Read the model definition and answer for the solid it produces. Units are mm, in the model's axes. A direction names the side the tool comes from. Give positions to 0.01 mm unless a question says otherwise; leave off trailing zeros. Write each loop counter-clockwise with the first axis right and the second up, starting at its lowest first coordinate (ties: lowest second). Pieces come first, ordered by that corner, then holes. Notation, with made-up numbers: (-39, 6.25) -> (-32, 6.25) arc R24 ccw to (-32, 19.25) -> close; hole circle Ø1 at (12.25, 33). An arc over 180 degrees is marked (long way). Write item = value, one per line.
from build123d import *

# Parameters (mm, degrees)
BOSS_EXTRUDE1_DEPTH = 5
BOSS_EXTRUDE2_DEPTH = 5


with BuildPart() as part:
    # Sketch1 → Boss-Extrude1 (new body)
    with BuildSketch(Plane(origin=(0, 0, 0), x_dir=(1, 0, 0), z_dir=(0, 1, 0))):
        Polygon((-109.888174915, 15), (-130.65513844, 15), (-130.65513844, 0), (-102.893560042, 0), align=None)
        Polygon((-98.854395725, 15), (-109.888174915, 15), (-102.893560042, 0), (-91.859780853, 0), align=None)
        Polygon((-91.859780853, 15), (-98.854395725, 15), (-91.859780853, 0), (-84.86516598, 0), align=None)
        Polygon((-80.826001663, 15), (-91.859780853, 15), (-84.86516598, 0), (-73.831386791, 0), align=None)
        Polygon((1.48976704, 15), (-80.826001663, 15), (-73.831386791, 0), (1.48976704, 0), align=None)
    extrude(amount=-BOSS_EXTRUDE1_DEPTH)

    # Sketch1_3 → Boss-Extrude2 (add)
    with BuildSketch(Plane(origin=(0, 0, 0), x_dir=(1, 0, 0), z_dir=(0, 1, 0))):
        Polygon((-109.888174915, 15), (-130.65513844, 15), (-130.65513844, 0), (-102.893560042, 0), align=None)
        Polygon((-91.859780853, 15), (-98.854395725, 15), (-91.859780853, 0), (-84.86516598, 0), align=None)
        Polygon((1.48976704, 15), (-80.826001663, 15), (-73.831386791, 0), (1.48976704, 0), align=None)
    extrude(amount=BOSS_EXTRUDE2_DEPTH)


solid = part.part
(1) Consider L1, parallel to X at y = 2.25, z = -2.75; L2, parallel to X at y = 3.75, z = -0.75; L3, parallel to Y at x = -99, z = -13.75. Determine where each line is inside the solid, lowest interval first.
Checks:
L1 = -130.66 to -104.18, -93.14 to -86.15, -75.11 to 1.49
L2 = -130.66 to -103.24, -92.21 to -85.21, -74.18 to 1.49
L3 = -5 to 0
(2) A tool of negligible diameter and unlimited length cuts with its end or side. For faces 4 (the flat face through (-83, 0, -8)), 5 (the flat face through (-64, 0, -15)), 6 (the flat face through (-77.378, 2.465, -7.605)), 7 (the flat face through (-106.342, 2.465, -7.395)), from which of +Z, -Z, +X, -X, +Y, -Y can it reach the whole face along a straight path? Write none if from no direction.
Checks:
face_4 = +Y
face_5 = -Z, +X, -X, +Y, -Y
face_6 = +Z, +Y
face_7 = -Z, +Y
(3) For a pull along X with two mould halves and no side action, classify faces 1 (the flat face through (-95.406, 2.465, -7.605)), 2 (the flat face through (-40, 5, -8)), 3 (the flat face through (-130.655, 0, -8)) as released by +X, released by -X, zero draft, split by the parting line, or undercut.
Checks:
face_1 = undercut
face_2 = zero draft
face_3 = released by -X
(4) The part is cut by section B-B on x = -77. Determine the outline of the cut face in (y, z), plus the area to 3 significant figures.
Checks:
outline = (-5, -15) -> (5, -15) -> (5, -6.8) -> (0, -6.8) -> (0, 0) -> (-5, 0) -> close
area = 116 mm²
(5) Given P1, Ø6, axis at x = -87, y = 3.5, coming from the -Z side, flat-ended and moving along its own axis, determine where the tip first touches the part or whether it passes through.
Checks:
P1 = -11.01
(6) The part is cut by section A-A on z = -6.75. Determine the outline of the cut face in (x, y), plus the area to 3 significant figures.
Checks:
outline = (-130.66, -5) -> (1.49, -5) -> (1.49, 5) -> (-76.98, 5) -> (-76.98, 0) -> (-88.01, 0) -> (-88.01, 5) -> (-95.01, 5) -> (-95.01, 0) -> (-106.04, 0) -> (-106.04, 5) -> (-130.66, 5) -> close
area = 1,210 mm²
